The listing builds one solid part. Answer for the finished solid, in the listing's coordinates (mm). A direction names the side the tool comes from. Coordinates: 2 decimals unless noted, no trailing zeros. Order: outer loops, then holes, each group sorted by start corner. A loop starts at its lowest first (then second) coordinate and runs counter-clockwise, first axis right, second up. Notation, with made-up numbers: (9, 89) -> (54, 89) arc R26 ccw to (54, 110) -> close; hole circle Ø3 at (59.25, 68). An arc over 180 degrees is marked (long way). Return JSON: item names as keys, results as strings.
Autodesk Inventor part; units mm, degrees
ref_plane "YZ Plane" through (0, 0, 0) normal (1, 0, 0) x (0, 1, 0)
ref_plane "XZ Plane" through (0, 0, 0) normal (0, 1, 0) x (-1, 0, 0)
ref_plane "XY Plane" through (0, 0, 0) normal (0, 0, 1) x (1, 0, 0)
sketch "Sketch1" plane through (0, 0, 0) normal (0, 0, 1) x (1, 0, 0)
  circle A0 centre (0, 0) radius 3.9624
  dimension "d0" = 7.9248
extrude "Extrusion1" add sketch "Sketch1" along normal blind 4.826
sketch "Sketch2" plane through (0, 0, 0) normal (0, 0, -1) x (-1, 0, 0)
  circle A0 centre (0, 0) radius 3.9624
  circle A1 centre (0, 0) radius 2.413
  dimension "d3" = 4.826
extrude "Extrusion2" add sketch "Sketch2" along normal blind 9.525 contours A1
sketch "Sketch3" plane through (0, 0, 4.826) normal (0, 0, 1) x (1, 0, 0)
  circle A0 centre (0, 0) radius 3.9624
  line L0 (-1.1457, 1.9844) -> (1.1457, 1.9844)
  line L1 (1.1457, 1.9844) -> (2.2914, 0)
  line L2 (2.2914, 0) -> (1.1457, -1.9844)
  line L3 (1.1457, -1.9844) -> (-1.1457, -1.9844)
  line L4 (-1.1457, -1.9844) -> (-2.2914, 0)
  line L5 (-2.2914, 0) -> (-1.1457, 1.9844)
  dimension "d6" = 3.9688
extrude "Extrusion3" cut sketch "Sketch3" against normal blind 3.175 contours L0 L1 L2 L3 L4 L5
thread "Thread1"
chamfer "Chamfer1" distance 0.508 angle 45 1 edges at (2.413, 0, -9.525)
chamfer "Chamfer2" distance 0.508 angle 45 1 edges at (-3.9624, 0, 4.826)
properties part number "10-32 x1000" material "Steel"
1. For faces 1 (the face through (0, -1.984, 3)), 2 (the face through (-2, -1, 4.826)), 3 (the face through (1.915, 1.468, -4.445)), determine the directions among +Z, -Z, +X, -X, +Y, -Y from which every point of the face is accessible in a straight line to the end or side of a thin tool.
Answer block:
{"face 1": "+Z", "face 2": "+Z, +X, -X, +Y, -Y", "face 3": "-Z"}
2. Each of these flat-tipped pins is pushed along its axis until it touches: pin 1 Ø4.5 at (x, y) = (1, 1) entering from +Z; pin 2 Ø3 at (y, z) = (-0.5, -7.5) entering from +X; pin 3 Ø4 at (x, z) = (-0.5, -8) entering from +Y. Where does it stop, or does it pass through?
Answer block:
{"pin 1": "stops at z = 4.83", "pin 2": "stops at x = 2.41", "pin 3": "stops at y = 2.41"}
3. The part is cut by section A-A on z = 2.5. Give the vertices of the cut face in (x, y).
Answer block:
{"outline": "circle Ø7.92 at (0, 0); hole (-2.29, 0) -> (-1.15, -1.98) -> (1.15, -1.98) -> (2.29, 0) -> (1.15, 1.98) -> (-1.15, 1.98) -> close"}
4. The part is cut by section B-B on x = 0. Give the vertices of the cut face in (y, z) (3 decimals), and give its area (3 significant figures).
Answer block:
{"outline": "(-3.962, 0) -> (-2.413, 0) -> (-2.413, -9.017) -> (-1.905, -9.525) -> (1.905, -9.525) -> (2.413, -9.017) -> (2.413, 0) -> (3.962, 0) -> (3.962, 4.318) -> (3.454, 4.826) -> (1.984, 4.826) -> (1.984, 1.651) -> (-1.984, 1.651) -> (-1.984, 4.826) -> (-3.454, 4.826) -> (-3.962, 4.318) -> close", "area": "71.1 mm2"}
5. The part is cut by section C-C on z = -2.5. Give the vertices of the cut face in (x, y).
Answer block:
{"outline": "circle Ø4.83 at (0, 0)"}
6. Consider line 1 (Y direction, x = -1.25, z = 3.5); line 2 (Z direction, x = 2.25, y = -1.5); line 3 (X direction, y = -1.5, z = 4.25). Determine where each line is inside the solid, lowest interval first. Write a range as from..to.
Answer block:
{"line 1": "y = -3.76..-1.8, 1.8..3.76", "line 2": "z = 0..4.83", "line 3": "x = -3.67..-1.43, 1.43..3.67"}
7. Determine the mould class of faces 4 (the face through (-0.52, -3.93, 2.13)), 5 (the face through (0, 0, -9.525)), 6 (the face through (-1.71, -1.01, 3.26)) for opening direction Y: pulls with the +Y half, pulls with the -Y half, needs draft (parallel to the pull), parting line crosses it, or undercut.
Answer block:
{"face 4": "parting line crosses it", "face 5": "needs draft", "face 6": "undercut"}
